from build123d import *

# Parameters (mm, degrees)
SCHIZZO1_R                    = 17
SCHIZZO1_R_2                  = 2.5
ESTRUSIONE_ESTRUSIONE2_DEPTH  = 20
M5_TAPPED_HOLE1_D             = 4.2
M5_TAPPED_HOLE1_DEPTH         = 17.4
M5_TAPPED_HOLE1_TIP           = 1.2618073
CBORE_FOR_M5_SHCS1_AT_2_COUNT = 2
CBORE_FOR_M5_SHCS1_AT_2_PITCH = 53
CBORE_FOR_M5_SHCS1_AT_3_COUNT = 2
CBORE_FOR_M5_SHCS1_AT_3_PITCH = 66.400301204
CBORE_FOR_M5_SHCS1_AT_4_COUNT = 2
CBORE_FOR_M5_SHCS1_AT_4_PITCH = 40
M6_TAPPED_HOLE1_D             = 5
M6_TAPPED_HOLE1_DEPTH         = 19
M6_TAPPED_HOLE1_TIP           = 1.502151548
CUT_EXTRUDE1_DEPTH            = 420.801540473


with BuildPart() as part:
    # Schizzo1 → Estrusione-Estrusione2 (new body)
    with BuildSketch(Plane.XY):
        with BuildLine():
            Line((5, 0), (95.262794416, 0))
            ThreePointArc((95.262794416, 0), (97.762794416, 0.669872981), (99.592921435, 2.5))
            Line((99.592921435, 2.5), (230.270234695, 228.839745962))
            ThreePointArc((230.270234695, 228.839745962), (230.769736807, 230.045650737), (230.940107676, 231.339745962))
            Line((230.940107676, 231.339745962), (230.940107676, 348))
            ThreePointArc((230.940107676, 348), (230.354321238, 349.414213562), (228.940107676, 350))
            Line((228.940107676, 350), (173.205080757, 350))
            ThreePointArc((173.205080757, 350), (163.205080757, 347.320508076), (155.884572681, 340))
            Line((155.884572681, 340), (0.669872981, 71.160254038))
            ThreePointArc((0.669872981, 71.160254038), (0.170370869, 69.954349263), (0, 68.660254038))
            Line((0, 68.660254038), (0, 5))
            ThreePointArc((0, 5), (1.464466094, 1.464466094), (5, 0))
        make_face()
        with Locations((208.940107676, 290)):
            Circle(SCHIZZO1_R, mode=Mode.SUBTRACT)
        with Locations((223.789350081, 304.849242405)):
            Circle(SCHIZZO1_R_2, mode=Mode.SUBTRACT)
        with Locations((223.789350081, 275.150757595)):
            Circle(SCHIZZO1_R_2, mode=Mode.SUBTRACT)
        with Locations((194.090865271, 275.150757595)):
            Circle(SCHIZZO1_R_2, mode=Mode.SUBTRACT)
        with Locations((194.090865271, 304.849242405)):
            Circle(SCHIZZO1_R_2, mode=Mode.SUBTRACT)
    extrude(amount=-ESTRUSIONE_ESTRUSIONE2_DEPTH)

    # M5 Tapped Hole1
    with Locations(Plane(origin=(50.131397208, 0, -10), x_dir=(0, 0, -1), z_dir=(0, -1, 0))):
        with Locations((0, 0), (0, 35), (0, -35)):
            Hole(M5_TAPPED_HOLE1_D / 2, depth=M5_TAPPED_HOLE1_DEPTH)
            with Locations((0, 0, -(M5_TAPPED_HOLE1_DEPTH + M5_TAPPED_HOLE1_TIP / 2))):  # 118° drill point
                Cone(0, M5_TAPPED_HOLE1_D / 2, M5_TAPPED_HOLE1_TIP, mode=Mode.SUBTRACT)

    # Sketch5 → CBORE for M5 SHCS1 (revolve, cut)
    with BuildSketch(Plane(origin=(80, 88.5, 0), x_dir=(0, -1, 0), z_dir=(1, 0, 0))):
        Polygon((0, 0), (0, 20), (2.65, 20), (2.65, 5), (5, 5), (5, 1.145), (6.145, 0), align=None)
    cbore_for_m5_shcs1 = revolve(axis=Axis((80, 88.5, 6.35), (0, 0, -1)), mode=Mode.SUBTRACT)

    # CBORE for M5 SHCS1 at 2: CBORE for M5 SHCS1 ×2
    with Locations(*[(0, -i * CBORE_FOR_M5_SHCS1_AT_2_PITCH, 0) for i in range(1, CBORE_FOR_M5_SHCS1_AT_2_COUNT)]):
        add(cbore_for_m5_shcs1, mode=Mode.SUBTRACT)

    # CBORE for M5 SHCS1 at 3: CBORE for M5 SHCS1 ×2
    with Locations(*[Vector(-0.6024069059118463, -0.7981891503332503, 0) * (i * CBORE_FOR_M5_SHCS1_AT_3_PITCH) for i in range(1, CBORE_FOR_M5_SHCS1_AT_3_COUNT)]):
        add(cbore_for_m5_shcs1, mode=Mode.SUBTRACT)

    # CBORE for M5 SHCS1 at 4: CBORE for M5 SHCS1 ×2
    with Locations(*[(-i * CBORE_FOR_M5_SHCS1_AT_4_PITCH, 0, 0) for i in range(1, CBORE_FOR_M5_SHCS1_AT_4_COUNT)]):
        add(cbore_for_m5_shcs1, mode=Mode.SUBTRACT)

    # M6 Tapped Hole1
    with Locations(Plane(origin=(230.940107676, 340, -10), x_dir=(0, 0, 1), z_dir=(1, 0, 0))):
        with Locations((0, 0), (0, 25), (0, 50), (0, 75), (0, 100)):
            Hole(M6_TAPPED_HOLE1_D / 2, depth=M6_TAPPED_HOLE1_DEPTH)
            with Locations((0, 0, -(M6_TAPPED_HOLE1_DEPTH + M6_TAPPED_HOLE1_TIP / 2))):  # 118° drill point
                Cone(0, M6_TAPPED_HOLE1_D / 2, M6_TAPPED_HOLE1_TIP, mode=Mode.SUBTRACT)

    # Sketch19 → Cut-Extrude1 (cut, through all)
    with BuildSketch(Plane.XY):
        with BuildLine():
            Line((180.542189015, 246.193907945), (188.198701931, 259.092660209))
            ThreePointArc((188.198701931, 259.092660209), (191.624579461, 259.966366767), (192.498286019, 256.540489237))
            Line((192.498286019, 256.540489237), (184.841773104, 243.641736973))
            ThreePointArc((184.841773104, 243.641736973), (181.415895574, 242.768030415), (180.542189015, 246.193907945))
        make_face()
        with BuildLine():
            Line((192.742918802, 200.660164494), (200.399431717, 213.558916758))
            ThreePointArc((200.399431717, 213.558916758), (203.825309247, 214.432623316), (204.699015805, 211.006745786))
            Line((204.699015805, 211.006745786), (197.04250289, 198.107993522))
            ThreePointArc((197.04250289, 198.107993522), (193.61662536, 197.234286964), (192.742918802, 200.660164494))
        make_face()
        with BuildLine():
            Line((147.20917535, 188.259881903), (154.865688266, 201.158634167))
            ThreePointArc((154.865688266, 201.158634167), (158.291565796, 202.032340725), (159.165272354, 198.606463195))
            Line((159.165272354, 198.606463195), (151.508759438, 185.707710931))
            ThreePointArc((151.508759438, 185.707710931), (148.082881908, 184.834004373), (147.20917535, 188.259881903))
        make_face()
        with BuildLine():
            Line((135.008445564, 233.993178159), (142.66495848, 246.891930423))
            ThreePointArc((142.66495848, 246.891930423), (146.09083601, 247.765636981), (146.964542568, 244.339759451))
            Line((146.964542568, 244.339759451), (139.308029652, 231.441007187))
            ThreePointArc((139.308029652, 231.441007187), (135.882152122, 230.567300629), (135.008445564, 233.993178159))
        make_face()
    extrude(amount=-CUT_EXTRUDE1_DEPTH, mode=Mode.SUBTRACT)


solid = part.part
Check sheet for the modelled part. Datum: model origin and axes. Units: mm. A direction names the side the tool comes from. Round coordinates to 2 decimals unless told otherwise and drop trailing zeros. Order: outer loops, then holes, each group sorted by start corner. A loop starts at its lowest first (then second) coordinate and runs counter-clockwise, first axis right, second up.
Q1. Cross-section at A-A, the plane x = 119. Enter the section's corners in (y, z).
Filled sheet:
outline: (36.11, -20) - (276.11, -20) - (276.11, 0) - (36.11, 0) - close
Q2. Depth check by flat-ended pin: P1, Ø5, axis at x = 80, y = 88.5, coming from the -Z side; P2, Ø2, axis at x = 84.5, z = -10, coming from the -Y side; P3, Ø4, axis at x = 122, z = -3.5, coming from the +Y side; P4, Ø1.5, axis at x = 60, z = -11, coming from the +Y side. Enter the tip coordinate at first touch or a pass-through.
Filled sheet:
P1: passes through
P2: stops at y = 17.68
P3: stops at y = 284.77
P4: stops at y = 175.22
Q3. Draft check along X on faces 1 (the face through (184.317, 252.553, -9.86)), 2 (the face through (164.02, 114.09, -9.86)), 3 (the face through (79.364, 207.462, -9.86)), 4 (the face through (42, 38, -5)). Enter one of: pulls with the +X half, pulls with the -X half, needs draft (parallel to the pull), parting line crosses it, or undercut.
Filled sheet:
face 1: undercut
face 2: pulls with the +X half
face 3: pulls with the -X half
face 4: undercut
Q4. Scan lines: L1, parallel to Y at x = 219.25, z = -10; L2, parallel to Z at x = 227, y = 290; L3, parallel to Y at x = 44, z = -4. Record each from-to range of solid material in increasing order.
Filled sheet:
L1: y = 209.75 to 237.5, 242.5 to 262.5, 267.5 to 276.48, 303.52 to 312.5, 317.5 to 337.5, 342.5 to 350
L2: z = -20 to -12.5, -7.5 to 0
L3: y = 0 to 32.5, 38.5 to 85.5, 91.5 to 146.21
Q5. Cross-section at B-B, the plane y = 219. Enter the section's corners in (x, z), plus the area to 3 significant figures.
Filled sheet:
outline: (86.03, -20) - (224.59, -20) - (224.59, 0) - (86.03, 0) - close
area: 2,770 mm2
Q6. Set-up check for faces 5 (the face through (49, 0, -12)), 6 (the face through (38.5, 83.73, -3.05)), 7 (the face through (188.724, 250.181, -9.86)): record each of +Z, -Z, +X, -X, +Y, -Y from which the full face is reachable in a straight line by a thin tool's end or side.
Filled sheet:
face 5: +Z, -Z, +X, -X, -Y
face 6: +Z
face 7: +Z, -Z
